Can you work these out from the drawing? Everything is in mm from the part's minimum corner. Give positions to 0.01 mm unless a question says otherwise; leave off trailing zeros. Order: outer loops, then holes, each group sorted by start corner. A loop starts at its lowest first (then second) coordinate and runs counter-clockwise, first axis right, second up. Notation, with made-up numbers: M 36,38 L 83,38 A28 cw 83,72 Z; hole C 43.5,45 d2. An arc over 180 degrees is marked long. Use a Markdown table: item, result. Add a question column.
Item 1: Suppose I cut it at A-A on x = 25.4. Write out the boundary of the cut face in (y, z).
Item 2: If I drill on L1, parallel to Z at x = 25.4, y = 3.5; L2, parallel to X at y = 8.25, z = 26; L3, parallel to Z at x = 33, y = 9.25, over which ranges is the centre line in solid material (lowest first)? Write a range as from..to.
Item 3: Suppose I cut it at C-C on y = 2.5. Write out the boundary of the cut face in (x, z), plus the area to 3 significant figures.
Item 4: If we mould it in two halves opening along X, with no side actions, what happens to the marked faces 1, 2 and 3? For each: released by +X, released by -X, zero draft, split by the parting line, or undercut.
Item 5: Suppose I cut it at B-B on z = 24. Write out the boundary of the cut face in (x, y).
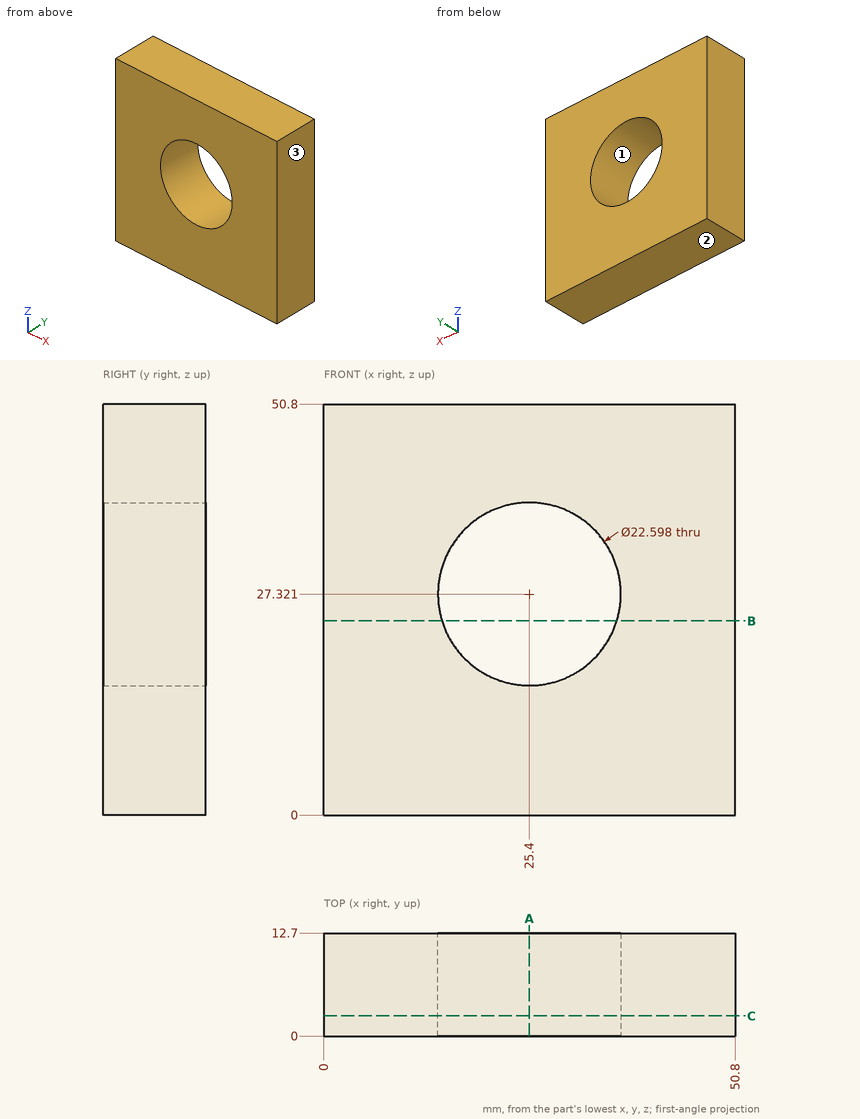
Findings below:
| question | item | result |
|---|---|---|
| 1 | outline | M 0,0 L 12.7,0 L 12.7,16.02 L 0,16.02 Z; M 0,38.62 L 12.7,38.62 L 12.7,50.8 L 0,50.8 Z |
| 2 | L1 | z = 0..16.02, 38.62..50.8 |
| 2 | L2 | x = 0..14.18, 36.62..50.8 |
| 2 | L3 | z = 0..18.96, 35.68..50.8 |
| 3 | outline | M 0,0 L 50.8,0 L 50.8,50.8 L 0,50.8 Z; hole C 25.4,27.32 d22.6 |
| 3 | area | 2,180 mm^2 |
| 4 | face 1 | undercut |
| 4 | face 2 | zero draft |
| 4 | face 3 | released by +X |
| 5 | outline | M 0,0 L 14.6,0 L 14.6,12.7 L 0,12.7 Z; M 36.2,0 L 50.8,0 L 50.8,12.7 L 36.2,12.7 Z |
